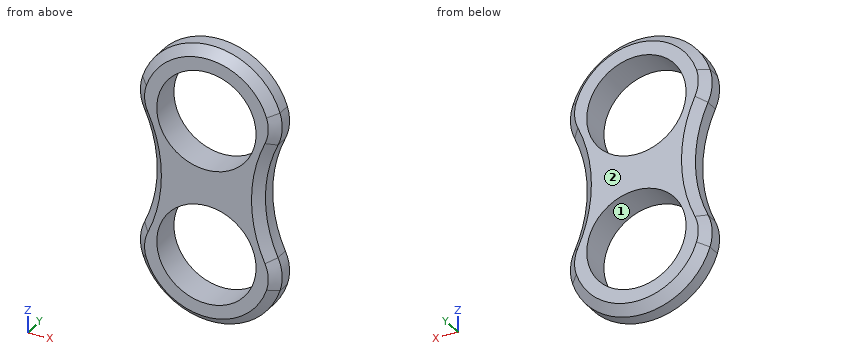
```python
from build123d import *

# Parameters (mm, degrees)
F0_R     = 11
F1_DEPTH = 7
F2_SIZE  = 2


with BuildPart() as f1:
    # F0 (on Front) → F1 (new body)
    with BuildSketch(Plane.XZ):
        with BuildLine():
            ThreePointArc((14.774496, 27.641957), (15.687594, 31.253782), (15.215308, 34.949181))
            ThreePointArc((15.215308, 34.949181), (0, 46), (-15.215308, 34.949181))
            ThreePointArc((-15.215308, 34.949181), (-15.687594, 31.253782), (-14.774496, 27.641957))
            ThreePointArc((-14.774496, 27.641957), (-11.980762, 15), (-14.774496, 2.358043))
            ThreePointArc((-14.774496, 2.358043), (-15.687594, -1.253782), (-15.215308, -4.949181))
            ThreePointArc((-15.215308, -4.949181), (0, -16), (15.215308, -4.949181))
            ThreePointArc((15.215308, -4.949181), (15.687594, -1.253782), (14.774496, 2.358043))
            ThreePointArc((14.774496, 2.358043), (11.980762, 15), (14.774496, 27.641957))
        make_face()
        Circle(F0_R, mode=Mode.SUBTRACT)
        with Locations((0, 30)):
            Circle(F0_R, mode=Mode.SUBTRACT)
    extrude(amount=F1_DEPTH)

    # F2
    f2_edges = [f1.edges().sort_by_distance(p)[0] for p in [
        (0, -7, 46),
        (0, 0, 46),
    ]]
    chamfer(f2_edges, length=F2_SIZE)


solid = f1.part
```
The listing builds one solid part. Answer for the finished solid, in the listing's coordinates (mm). Face numbers are marked on the shaded views. Round coordinates to 2 decimals unless told otherwise and drop trailing zeros. Write each loop counter-clockwise with the first axis right and the second up, starting at its lowest first coordinate (ties: lowest second). Pieces come first, ordered by that corner, then holes. Notation, with made-up numbers: (-23, -11) -> (19, -11) arc R11 cw to (19, 0) -> close; hole circle Ø4 at (-2, 22). An arc over 180 degrees is marked (long way). Answer as a JSON object with one key per item and string values. Group by question number.
Q1. Each of these flat-tipped pins is pushed along its axis until it touches: pin 1 Ø4 at (y, z) = (-5.5, 12.5) entering from +X; pin 2 Ø10 at (x, z) = (-12, 20.5) entering from +Y; pin 3 Ø4 at (x, y) = (-5, -6) entering from +Z; pin 4 Ø1 at (y, z) = (-2.5, -9.5) entering from -X. Where does it stop, or does it pass through?
Q2. Section A-A (x = 0) is taken. Write down the section's boundary in (y, z).
Q3. Section B-B (x = 4.5) is taken. Count the separate pieces of the cut face and the enclosed holes in it, plus the area to 3 significant figures.
Q4. Straight lines are drawn through the part: line 1 along Z through (x, y) = (-7.5, -1.75); line 2 along Z through (x, y) = (-3.5, -5.5); line 3 along X through (y, z) = (-3.75, -8.5). For each, find the intervals that lie inside material, in ascending order.
Q5. Determine the mould class of the marked faces 1 and 2 for opening direction Z: pulls with the +Z half, pulls with the -Z half, needs draft (parallel to the pull), parting line crosses it, or undercut.
Check values:
{
 "1": {"pin 1": "x = 12.31", "pin 2": "y = 0", "pin 3": "z = 45.66", "pin 4": "x = -13.23"},
 "2": {"outline": "(-7, -14) -> (-5, -16) -> (-2, -16) -> (0, -14) -> (0, -11) -> (-7, -11) -> close; (-7, 11) -> (0, 11) -> (0, 19) -> (-7, 19) -> close; (-7, 41) -> (0, 41) -> (0, 44) -> (-2, 46) -> (-5, 46) -> (-7, 44) -> close"},
 "3": {"separate pieces": "3", "enclosed holes": "0", "area": "136 mm^2"},
 "4": {"line 1": "-13.85 to -8.05, 8.05 to 21.95, 38.05 to 43.85", "line 2": "-15.1 to -10.43, 10.43 to 19.57, 40.43 to 45.1", "line 3": "-13.56 to -6.98, 6.98 to 13.56"},
 "5": {"face 1": "undercut", "face 2": "needs draft"}
}
